from build123d import *

# Parameters (mm, degrees)
SKETCH1_W                        = 80
SKETCH1_H                        = 80
BOSS_EXTRUDE1_DEPTH              = 6
F_10_5_10_5_DIAMETER_HOLE1_D     = 10.5
F_10_5_10_5_DIAMETER_HOLE1_DEPTH = 6
CHAMFER1_SIZE                    = 5
CHAMFER2_SIZE                    = 1
FILLET1_R                        = 1
FILLET2_R                        = 2
SCALE1_SCALE                     = 0.75


with BuildPart() as part:
    # Sketch1 → Boss-Extrude1 (new body)
    with BuildSketch(Plane.XY.offset(6)):
        Rectangle(SKETCH1_W, SKETCH1_H)
    extrude(amount=-BOSS_EXTRUDE1_DEPTH)

    # Sketch2 → Revolve1 (revolve)
    with BuildSketch(Plane(origin=(0, 0, 0), x_dir=(1, 0, 0), z_dir=(0, 1, 0))):
        Polygon((25, -6), (0, -6), (0, -12), (22.816178594, -12), align=None)
    revolve(axis=Axis((0, 0, 6), (0, 0, 1)))

    # Sketch3 → Cut-Revolve1 (revolve, cut)
    with BuildSketch(Plane(origin=(0, 0, 0), x_dir=(1, 0, 0), z_dir=(0, 1, 0))):
        Polygon((26, 0), (0, 0), (0, -12), (18, -12), (18, -10.143593539), (22, -9.07179677), (22, -7.07179677), (18, -6), (18, -4), (26, -4), align=None)
    revolve(axis=Axis((0, 0, 0), (0, 0, 1)), mode=Mode.SUBTRACT)

    # Ø10.5 (10.5) Diameter Hole1
    with Locations(Plane.XY.offset(6)):
        with Locations((30, 30), (-30, 30), (-30, -30), (30, -30)):
            Hole(F_10_5_10_5_DIAMETER_HOLE1_D / 2, depth=F_10_5_10_5_DIAMETER_HOLE1_DEPTH)

    # Chamfer1
    chamfer1_edges = [part.edges().sort_by_distance(p)[0] for p in [
        (-40, -40, 3),
        (-40, 40, 3),
        (40, 40, 3),
        (40, -40, 3),
    ]]
    chamfer(chamfer1_edges, length=CHAMFER1_SIZE)

    # Chamfer2
    chamfer2_edges = [part.edges().sort_by_distance(p)[0] for p in [
        (-26, 0, 0),
        (35.25, -30, 6),
        (-24.75, -30, 6),
        (-24.75, 30, 6),
        (35.25, 30, 6),
    ]]
    chamfer(chamfer2_edges, length=CHAMFER2_SIZE)

    # Fillet1
    fillet1_edges = [part.edges().sort_by_distance(p)[0] for p in [
        (-26, 0, 4),
    ]]
    fillet(fillet1_edges, radius=FILLET1_R)

    # Fillet2
    fillet2_edges = [part.edges().sort_by_distance(p)[0] for p in [
        (-25, 0, 6),
    ]]
    fillet(fillet2_edges, radius=FILLET2_R)


with BuildPart() as part_1:
    # Scale1: scaled about (0, 0, 3.839535201)
    add(part.part.scale(SCALE1_SCALE).moved(Location((0, 0, 0.9598838))))


solid = part_1.part
Read the model definition and answer for the solid it produces. Units are mm, in the model's axes. A direction names the side the tool comes from. Round coordinates to 2 decimals unless told otherwise and drop trailing zeros. Order: outer loops, then holes, each group sorted by start corner. A loop starts at its lowest first (then second) coordinate and runs counter-clockwise, first axis right, second up.
1) Flat-ended cylindrical pins translate along their axes: pin 1 (2 mm diameter, centred on x = -3.5, z = 8.5, fed in from -Y); pin 2 (4 mm diameter, centred on x = 7.5, y = 12, fed in from -Z). Find the tip coordinate at first contact, or state that the pin passes through.
2) The part is cut by section A-A on y = 22.5. Write down the section's boundary in (x, z).
3) Straight lines are drawn through the part: L1, parallel to Y at x = -22.5, z = 2.95; L2, parallel to Z at x = 17, y = -17.5; L3, parallel to Y at x = 12, z = 2.5. For each, find the intervals that lie inside material, in ascending order.
4) For faces 5 (the face through (-2.539, 19.334, 2.449)), 6 (the face through (-0.4, 20.4, 0.96)), 7 (the face through (0, 20, 5.46)), determine the directions among +Z, -Z, +X, -X, +Y, -Y from which every point of the face is accessible in a straight line to the end or side of a thin tool.
5) The mould has two halves that part along X. Classify faces 1 (the face through (13.056, 4.111, 8.517)), 2 (the face through (0, 30, 3)), 3 (the face through (30, 0, 3)), 4 (the face through (-19.38, 20.1, 2.81)): released by +X, released by -X, zero draft, split by the parting line, or undercut.
Resolved:
1. pin 1: stops at y = -17.71
1. pin 2: stops at z = 3.96
2. outline: (-30, 0.96) - (-26.44, 0.96) - (-26.44, 4.71) - (-27.19, 5.46) - (-30, 5.46) - close; (-18.56, 0.96) - (18.56, 0.96) - (18.56, 4.71) - (17.81, 5.46) - (-17.81, 5.46) - (-18.56, 4.71) - close; (26.44, 0.96) - (30, 0.96) - (30, 5.46) - (27.19, 5.46) - (26.44, 4.71) - close
3. L1: y = -30 to -26.44, -18.56 to 18.56, 26.44 to 30
3. L2: z = 0.96 to 5.46
3. L3: y = -30 to -15.37, 15.37 to 30
4. face 5: -Z
4. face 6: -Z, +X, -X, +Y, -Y
4. face 7: +Z
5. face 1: undercut
5. face 2: zero draft
5. face 3: released by +X
5. face 4: undercut
